```python
from build123d import *

# Parameters (mm, degrees)
SKETCH1_W           = 80.01
SKETCH1_H           = 80.01
BOSS_EXTRUDE1_DEPTH = 24.638
SKETCH2_R           = 38.735
SKETCH2_R_2         = 2.159
CUT_EXTRUDE1_DEPTH  = 24.638
FILLET1_R           = 2.54
BOSS_EXTRUDE2_DEPTH = 2.54


with BuildPart() as part:
    # Sketch1 → Boss-Extrude1 (new body)
    with BuildSketch(Plane(origin=(0, 0, 0), x_dir=(1, 0, 0), z_dir=(0, 1, 0))):
        Rectangle(SKETCH1_W, SKETCH1_H)
    extrude(amount=BOSS_EXTRUDE1_DEPTH)

    # Sketch2 → Cut-Extrude1 (cut)
    with BuildSketch(Plane(origin=(0, 24.638, 0), x_dir=(1, 0, 0), z_dir=(0, 1, 0))):
        with Locations(Location((0, 0, 0), (0, 0, 270))):
            Circle(SKETCH2_R)
        with Locations(Location((-36.068, 36.068, 0), (0, 0, 270))):
            Circle(SKETCH2_R_2)
        with Locations(Location((36.068, 36.068, 0), (0, 0, 270))):
            Circle(SKETCH2_R_2)
        with Locations(Location((36.068, -36.068, 0), (0, 0, 270))):
            Circle(SKETCH2_R_2)
        with Locations(Location((-36.068, -36.068, 0), (0, 0, 270))):
            Circle(SKETCH2_R_2)
    extrude(amount=-CUT_EXTRUDE1_DEPTH, mode=Mode.SUBTRACT)

    # Fillet1
    fillet1_edges = [part.edges().sort_by_distance(p)[0] for p in [
        (40.005, 12.319, 40.005),
        (-40.005, 12.319, 40.005),
        (-40.005, 12.319, -40.005),
        (40.005, 12.319, -40.005),
    ]]
    fillet(fillet1_edges, radius=FILLET1_R)

    # Sketch3 → Boss-Extrude2 (add)
    with BuildSketch(Plane(origin=(0, 24.638, 0), x_dir=(1, 0, 0), z_dir=(0, 1, 0))):
        with BuildLine():
            Line((17.272, 0), (17.272, 34.671))
            ThreePointArc((17.272, 34.671), (16.01238371, 35.270437946), (14.732, 35.824131546))
            Line((14.732, 35.824131546), (14.732, 9.016105589))
            ThreePointArc((14.732, 9.016105589), (8.443808627, 15.067318271), (0, 17.272))
            Line((0, 17.272), (-34.671, 17.272))
            ThreePointArc((-34.671, 17.272), (-35.270437946, 16.01238371), (-35.824131546, 14.732))
            Line((-35.824131546, 14.732), (-9.016105589, 14.732))
            ThreePointArc((-9.016105589, 14.732), (-15.067318271, 8.443808627), (-17.272, 0))
            Line((-17.272, 0), (-17.272, -34.671))
            ThreePointArc((-17.272, -34.671), (-16.01238371, -35.270437946), (-14.732, -35.824131546))
            Line((-14.732, -35.824131546), (-14.732, -9.016105589))
            ThreePointArc((-14.732, -9.016105589), (-8.443808627, -15.067318271), (0, -17.272))
            Line((0, -17.272), (34.671, -17.272))
            ThreePointArc((34.671, -17.272), (35.270437946, -16.01238371), (35.824131546, -14.732))
            Line((35.824131546, -14.732), (9.016105589, -14.732))
            ThreePointArc((9.016105589, -14.732), (15.067318271, -8.443808627), (17.272, 0))
        make_face()
    extrude(amount=-BOSS_EXTRUDE2_DEPTH)


solid = part.part
```
The model under review builds one solid part; all positions refer to its coordinate system, in mm. A direction names the side the tool comes from. Coordinates: 2 decimals unless noted, no trailing zeros. Write each loop counter-clockwise with the first axis right and the second up, starting at its lowest first coordinate (ties: lowest second). Pieces come first, ordered by that corner, then holes. Notation, with made-up numbers: (79.25, 36.25) -> (110.25, 36.25) arc R29 cw to (110.25, 71.25) -> close; hole circle Ø11 at (-22, 69.25). An arc over 180 degrees is marked (long way). One line per item, written item: value. Start each with the question number.
Q1. Add section C-C, the plane y = 19.75. Give the boundary of the cut face in (x, z) (3 decimals).
Q2. Add section B-B, the plane x = 26.5. Give the boundary of the cut face in (y, z) (3 decimals).
Q3. Clearance check with flat-ended pins moving along their axes: P1, Ø2.5, axis at x = 36.068, z = 36.068, coming from the +Y side; P2, Ø21.5, axis at x = -17, z = -5, coming from the -Y side. State where each tip first meets the part, or that it passes through.
Q4. To check wall thickness, follow probe 1 along X at (y, z) = (4, 0.5) (3 decimals); probe 2 along Z at (x, y) = (-7.5, 1.5) (3 decimals); probe 3 along Y at (x, z) = (-16, 17). State the ranges of each line that lie inside material, in increasing order.
Q5. For faces 1 (the face through (-39.28, 12.49, 39.24)), 2 (the face through (17, 23, 17.272)), list the 3-axis set-ups (+Z, -Z, +X, -X, +Y, -Y) from which the entire face can be reached by the end or side of a thin tool; tool diameter is ignored.
Q6. Add section A-A, the plane z = 11. Give the boundary of the cut face in (x, y) (3 decimals), then the cut area to 3 significant figures.
Q7. The part is to be moulded in two halves that separate along Z. For faces 3 (the face through (-34.25, 12.49, 37.23)), 4 (the face through (-1, 12, 40.005)), 5 (the face through (-1, 24.638, -1)), say which applies: +Z half, -Z half, draft (parallel to the pull), parting line (faces both ways), or undercut.
Q8. Add section D-D, the plane z = 32.5. Give the boundary of the cut face in (x, y) (3 decimals).
Response:
1. outline: (-40.005, -37.465) arc R2.54 ccw to (-37.465, -40.005) -> (37.465, -40.005) arc R2.54 ccw to (40.005, -37.465) -> (40.005, 37.465) arc R2.54 ccw to (37.465, 40.005) -> (-37.465, 40.005) arc R2.54 ccw to (-40.005, 37.465) -> close; hole circle Ø77.47 at (0, 0); hole circle Ø4.318 at (-36.068, -36.068); hole circle Ø4.318 at (-36.068, 36.068); hole circle Ø4.318 at (36.068, -36.068); hole circle Ø4.318 at (36.068, 36.068)
2. outline: (0, -40.005) -> (24.638, -40.005) -> (24.638, -28.252) -> (0, -28.252) -> close; (0, 28.252) -> (24.638, 28.252) -> (24.638, 40.005) -> (0, 40.005) -> close; (22.098, 14.732) -> (24.638, 14.732) -> (24.638, 17.272) -> (22.098, 17.272) -> close
3. P1: through
3. P2: y = 22.1
4. probe 1: -40.005 to -38.732, 38.732 to 40.005
4. probe 2: -40.005 to -38.002, 38.002 to 40.005
4. probe 3: 22.1 to 24.64
5. face 1: +Z, -X, +Y, -Y
5. face 2: +Y, -Y
6. outline: (-40.005, 0) -> (-37.14, 0) -> (-37.14, 24.638) -> (-40.005, 24.638) -> close; (-17.272, 22.098) -> (-14.732, 22.098) -> (-14.732, 24.638) -> (-17.272, 24.638) -> close; (-13.316, 22.098) -> (13.316, 22.098) -> (13.316, 24.638) -> (-13.316, 24.638) -> close; (37.14, 0) -> (40.005, 0) -> (40.005, 24.638) -> (37.14, 24.638) -> close
6. area: 215 mm²
7. face 3: undercut
7. face 4: +Z half
7. face 5: draft
8. outline: (-40.005, 0) -> (-21.075, 0) -> (-21.075, 24.638) -> (-40.005, 24.638) -> close; (-17.272, 22.098) -> (-14.732, 22.098) -> (-14.732, 24.638) -> (-17.272, 24.638) -> close; (21.075, 0) -> (40.005, 0) -> (40.005, 24.638) -> (21.075, 24.638) -> close
